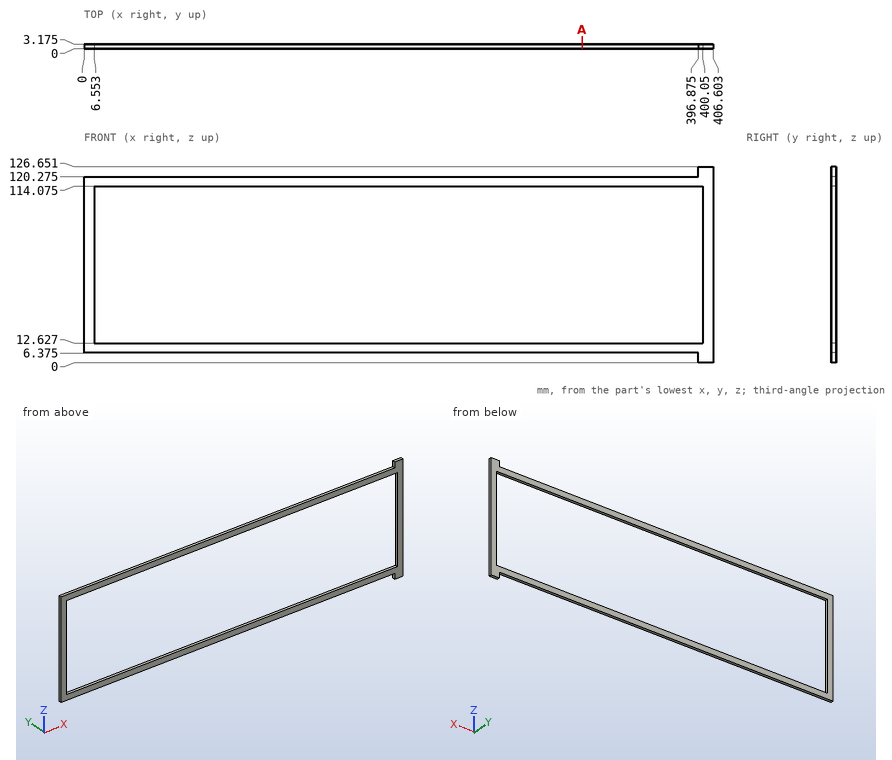
For this review, use the dimensioned drawing (mm, ordinates from the lowest corner) and the shaded views. Give positions to 0.01 mm unless a question says otherwise; leave off trailing zeros. Loops run counter-clockwise (first coordinate to the right, second up) from the corner with the lowest first, then second, coordinate; pieces in that order, holes last. Notation, with made-up numbers: (-1, -0.5) - (17, -0.5) arc R8 ccw to (17, 13.5) - close; hole circle Ø11 at (-19.5, -10.75). An arc over 180 degrees is marked (long way). Write each question's results on one line, items separated by ' | '.
(1) For pin 1 Ø1 at (x, y) = (279.5, 1.5) entering from +Z (1 decimal); pin 2 Ø1.6 at (x, y) = (159, 1) entering from -Z (1 decimal), all flat-tipped, find the tip position at first contact; note any pin that passes through.
Conclusion:
pin 1: z = 120.3 | pin 2: z = 6.4
(2) For line 1 along Z through (x, y) = (138, 1.75) (1 decimal); line 2 along X through (y, z) = (2.45, 39), list the stretches that pass through material, from the lowest coordinate up.
Conclusion:
line 1: 6.4 to 12.6, 114.1 to 120.3 | line 2: 0 to 6.55, 400.05 to 406.6
(3) Take a section at A-A (x = 322). Give the boundary of the cut face in (y, z) (1 decimal).
Conclusion:
outline: (0, 6.4) - (3.2, 6.4) - (3.2, 12.6) - (0, 12.6) - close; (0, 114.1) - (3.2, 114.1) - (3.2, 120.3) - (0, 120.3) - close
